```python
from build123d import *

# Parameters (mm, degrees)
ESQUISSE1_W             = 110
ESQUISSE1_H             = 140
ESQUISSE1_R             = 1.5
BOSS_EXTRU_1_DEPTH      = 5
ESQUISSE2_W             = 5
ESQUISSE2_H             = 140
BOSS_EXTRU_2_DEPTH      = 5
ESQUISSE3_R             = 10
ENL_V_MAT_EXTRU_1_DEPTH = 10


with BuildPart() as part:
    # Esquisse1 → Boss.-Extru.1 (new body)
    # profile 1 of 5: a face of its own
    with BuildSketch(Plane.XY):
        Rectangle(ESQUISSE1_W, ESQUISSE1_H)
    # profile 2 of 5: a face of its own
    with BuildSketch(Plane.XY):
        Polygon((-15, 70), (-55, 70), (-55, 15), (-55, -15), (-55, -70), (-15, -70), (15, -70), (55, -70), (55, -15), (55, 15), (55, 70), (15, 70), align=None)
    # profile 3 of 5: a face of its own
    with BuildSketch(Plane.XY):
        with BuildLine():
            Line((15, -70), (-15, -70))
            Line((-15, -70), (-15, -75))
            Line((-15, -75), (-1.658312395, -75))
            ThreePointArc((-1.658312395, -75), (0, -75.5), (1.658312395, -75))
            Line((1.658312395, -75), (15, -75))
            Line((15, -75), (15, -70))
        make_face()
        with Locations((0, -72.5)):
            Circle(ESQUISSE1_R, mode=Mode.SUBTRACT)
    # profile 4 of 5: a face of its own
    with BuildSketch(Plane.XY):
        with BuildLine():
            Line((60, 15), (55, 15))
            Line((55, 15), (55, -15))
            Line((55, -15), (60, -15))
            Line((60, -15), (60, -1.658312395))
            ThreePointArc((60, -1.658312395), (60.5, 0), (60, 1.658312395))
            Line((60, 1.658312395), (60, 15))
        make_face()
        with Locations((57.5, 0)):
            Circle(ESQUISSE1_R, mode=Mode.SUBTRACT)
    # profile 5 of 5: a face of its own
    with BuildSketch(Plane.XY):
        with BuildLine():
            Line((-15, 75), (-15, 70))
            Line((-15, 70), (15, 70))
            Line((15, 70), (15, 75))
            Line((15, 75), (1.658312395, 75))
            ThreePointArc((1.658312395, 75), (0, 75.5), (-1.658312395, 75))
            Line((-1.658312395, 75), (-15, 75))
        make_face()
        with Locations((0, 72.5)):
            Circle(ESQUISSE1_R, mode=Mode.SUBTRACT)
    extrude(amount=BOSS_EXTRU_1_DEPTH)

    # Esquisse2 → Boss.-Extru.2 (add)
    with BuildSketch(Plane.ZY.offset(55)):
        with Locations((2.5, 0)):
            Rectangle(ESQUISSE2_W, ESQUISSE2_H)
    extrude(amount=BOSS_EXTRU_2_DEPTH)

    # Esquisse3 → Enlèv. mat.-Extru.1 (cut)
    with BuildSketch(Plane.XY.offset(5)):
        with Locations((30, -50)):
            Circle(ESQUISSE3_R)
    extrude(amount=-ENL_V_MAT_EXTRU_1_DEPTH, mode=Mode.SUBTRACT)


solid = part.part
```
The model under review builds one solid part; all positions refer to its coordinate system, in mm. A direction names the side the tool comes from. Give positions to 0.01 mm unless a question says otherwise; leave off trailing zeros. Write each loop counter-clockwise with the first axis right and the second up, starting at its lowest first coordinate (ties: lowest second). Pieces come first, ordered by that corner, then holes. Notation, with made-up numbers: (89, -2) -> (128, -2) arc R27 cw to (128, 16) -> close; hole circle Ø4 at (52.5, -6). An arc over 180 degrees is marked (long way). Answer in a Markdown table with one row per item.
1) Add section A-A on y = -50. State the section outline as (x, z) points, plus the area to 3 significant figures.
Worked answers:
| item | result |
|---|---|
| outline | (-60, 0) -> (20, 0) -> (20, 5) -> (-60, 5) -> close; (40, 0) -> (55, 0) -> (55, 5) -> (40, 5) -> close |
| area | 475 mm² |
2) Add section C-C on x = -30. State the section outline as (y, z) points, plus the area to 3 significant figures.
Worked answers:
| item | result |
|---|---|
| outline | (-70, 0) -> (70, 0) -> (70, 5) -> (-70, 5) -> close |
| area | 700 mm² |
3) Clearance check with flat-ended pins moving along their axes: P1, Ø2.5, axis at y = -34.5, z = 3.5, coming from the +X side; P2, Ø1.5, axis at x = -20.5, z = 1, coming from the +Y side; P3, Ø1.5, axis at x = 58.5, z = 2.5, coming from the -Y side; P4, Ø2.5, axis at x = 57.5, y = 0, coming from the -Z side. State where each tip first meets the part, or that it passes through.
Worked answers:
| item | result |
|---|---|
| P1 | x = 55 |
| P2 | y = 70 |
| P3 | y = -15 |
| P4 | through |
4) Mouldability with a two-part tool opening along X and no side actions: class faces 4 (the flat face through (8, -75, 2)), 5 (the cylindrical face through (0.806, -71.235, 2.465)), 6 (the flat face through (60, 8, 2)) as +X half, -X half, draft (parallel to the pull), parting line (faces both ways), or undercut.
Worked answers:
| item | result |
|---|---|
| face 4 | draft |
| face 5 | undercut |
| face 6 | +X half |
5) Add section B-B on z = 1. State the section outline as (x, y) points, plus the area to 3 significant figures.
Worked answers:
| item | result |
|---|---|
| outline | (-60, -70) -> (-15, -70) -> (-15, -75) -> (-1.66, -75) arc R3 ccw to (1.66, -75) -> (15, -75) -> (15, -70) -> (55, -70) -> (55, -15) -> (60, -15) -> (60, -1.66) arc R3 ccw to (60, 1.66) -> (60, 15) -> (55, 15) -> (55, 70) -> (15, 70) -> (15, 75) -> (1.66, 75) arc R3 ccw to (-1.66, 75) -> (-15, 75) -> (-15, 70) -> (-60, 70) -> close; hole circle Ø3 at (0, -72.5); hole circle Ø3 at (0, 72.5); hole circle Ø20 at (30, -50); hole circle Ø3 at (57.5, 0) |
| area | 16,200 mm² |
6) For L1, parallel to X at y = 72.5, z = 3.65; L2, parallel to X at y = 10, z = 3.1; L3, parallel to X at y = 39.5, z = 3.05, list the stretches that pass through material, from the lowest coordinate up. Write a range as [from, to].
Worked answers:
| item | result |
|---|---|
| L1 | [-15, -1.5], [1.5, 15] |
| L2 | [-60, 60] |
| L3 | [-60, 55] |
7) Tool access review of faces 1 (the flat face through (-8, -75, 2)), 2 (the flat face through (57, -15, 2)), 3 (the flat face through (-8, 75, 2)): name each direction out of +Z, -Z, +X, -X, +Y, -Y from which nothing blocks a thin tool from reaching the whole face with its end or side.
Worked answers:
| item | result |
|---|---|
| face 1 | +Z, -Z, -X, -Y |
| face 2 | +Z, -Z, +X, -Y |
| face 3 | +Z, -Z, -X, +Y |
8) Add section D-D on y = 55. State the section outline as (x, z) points.
Worked answers:
| item | result |
|---|---|
| outline | (-60, 0) -> (55, 0) -> (55, 5) -> (-60, 5) -> close |
